Here's how the part is built. I have some questions about the finished solid (model axes, mm). Round coordinates to 2 decimals unless told otherwise and drop trailing zeros. Order: outer loops, then holes, each group sorted by start corner. A loop starts at its lowest first (then second) coordinate and runs counter-clockwise, first axis right, second up.
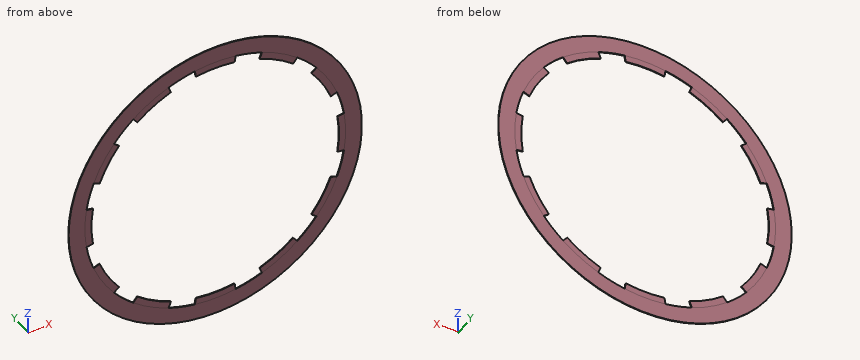
Autodesk Inventor part; units mm, degrees
ref_plane "YZ Plane" through (0, 0, 0) normal (1, 0, 0) x (0, 1, 0)
ref_plane "XZ Plane" through (0, 0, 0) normal (0, 1, 0) x (-1, 0, 0)
ref_plane "XY Plane" through (0, 0, 0) normal (0, 0, 1) x (1, 0, 0)
sketch "Sketch1" plane through (0, 0, 0) normal (0, 0, 1) x (1, 0, 0)
  line L0 (-20, 0) -> (-22.5, 0)
  line L1 (-22.5, 0) -> (-22.5, 0.1)
  line L2 (-22.5, 0.1) -> (-20, 0.1)
  line L3 (-20, 0.1) -> (-20, 0)
  line L4 (0, -0.02) -> (0, 0.12)
  point P0 (0, 0)
  dimension "d0" = 20
  dimension "d1" = 22.5
  dimension "d2" = 0.1
revolve "Revolution1" add sketch "Sketch1" angle 360 about axis through (0, -10, 0) along (0, 1, 0)
sketch "Sketch2" plane through (0, 0.1, 0) normal (0, 1, 0) x (1, 0, 0)
  circle A0 centre (0, 0) radius 19 construction
  line L0 (0, 0) -> (-19.7538, 3.1287)
  line L1 (0, 0) -> (-19.7538, -3.1287)
  circle A1 centre (0, 0) radius 20
  circle A2 centre (0, 0) radius 20
  arc A3 (-18.7661, 2.9723) -> (-18.7661, -2.9723) centre (0, 0) ccw
  arc A4 (-19.7538, 3.1287) -> (-19.7538, -3.1287) centre (0, 0) ccw
  point P0 (-19.7538, 3.1287)
  dimension "d4" = 38
  dimension "d5" = 18
extrude "Extrusion1" add sketch "Sketch2" against normal up to surface (0.1 mm away) contours A3 L1 A1 L0
pattern_circular "Circular Pattern1" count 12 over 360 about axis through (0, 0.05, 0) along (0, 1, 0) of "Extrusion1"
properties part number "TorsionOscillator-IsolationRing" material "Paper"
1) If we section it at A-A (z = 0): Write out the boundary of the cut face in (x, y).
2) If we section it at B-B (x = 0): Write out the boundary of the cut face in (y, z).
3) I need wall thicknesses on line 1 (X direction, y = 0.05, z = -1.5); line 2 (Z direction, x = -17, y = 0.05); line 3 (X direction, y = 0.05, z = 16). Which ranges of each line are inside material? Lowest first, please.
Solutions:
1. outline: (-22.5, 0) - (-19, 0) - (-19, 0.1) - (-22.5, 0.1) - close; (19, 0) - (22.5, 0) - (22.5, 0.1) - (19, 0.1) - close
2. outline: (0, -22.5) - (0.1, -22.5) - (0.1, -19) - (0, -19) - close; (0, 19) - (0.1, 19) - (0.1, 22.5) - (0, 22.5) - close
3. line 1: x = -22.45 to -18.94, 18.94 to 22.45
3. line 2: z = -14.74 to -8.49, 8.49 to 14.74
3. line 3: x = -15.82 to -10.25, 10.25 to 15.82
